Geometry: final body of the model. Coordinates: model frame, mm. A direction names the side the tool comes from. Coordinates: 2 decimals unless noted, no trailing zeros. Write each loop counter-clockwise with the first axis right and the second up, starting at its lowest first coordinate (ties: lowest second). Pieces come first, ordered by that corner, then holes.
from build123d import *

# Parameters (mm, degrees)
SKETCH1_W            = 68
SKETCH1_H            = 70
BOSS_EXTRUDE2_DEPTH  = 4
SKETCH2_W            = 13.5
SKETCH2_H            = 5
BOSS_EXTRUDE4_DEPTH  = 22
SKETCH3_R            = 2
CUT_EXTRUDE1_DEPTH   = 10
SKETCH4_W            = 5
SKETCH4_H            = 25.69
BOSS_EXTRUDE5_DEPTH  = 15
SKETCH5_R            = 1.3
CUT_EXTRUDE2_DEPTH   = 6
SKETCH6_W            = 68
SKETCH6_H            = 4
BOSS_EXTRUDE6_DEPTH  = 10
BOSS_EXTRUDE7_DEPTH  = 22
SKETCH8_W            = 3
SKETCH8_H            = 26
BOSS_EXTRUDE8_DEPTH  = 22
BOSS_EXTRUDE9_DEPTH  = 22
SKETCH12_W           = 3
SKETCH12_H           = 1
CUT_EXTRUDE5_DEPTH   = 7
SKETCH13_W           = 68
SKETCH13_H           = 26
SKETCH13_H_2         = 15
BOSS_EXTRUDE12_DEPTH = 8
SKETCH19_W           = 6
SKETCH19_H           = 61
CUT_EXTRUDE8_DEPTH   = 22
SKETCH20_W           = 3
SKETCH20_H           = 3
BOSS_EXTRUDE13_DEPTH = 22
SKETCH21_R           = 2.5
CUT_EXTRUDE9_DEPTH   = 22
SKETCH22_R           = 5.004310541
SKETCH22_R_2         = 5.00398022
SKETCH22_R_3         = 4.995044229
SKETCH22_R_4         = 4.998284189
CUT_EXTRUDE10_DEPTH  = 6
SKETCH24_W           = 3
SKETCH24_H           = 3
BOSS_EXTRUDE14_DEPTH = 22
SKETCH26_R           = 1.2
CUT_EXTRUDE11_DEPTH  = 5
SKETCH27_R           = 2.5
CUT_EXTRUDE13_DEPTH  = 10
FILLET2_R            = 2.5


with BuildPart() as part:
    # Sketch1 → Boss-Extrude2 (new body)
    with BuildSketch(Plane(origin=(0, 0, 0), x_dir=(1, 0, 0), z_dir=(0, 1, 0))):
        with Locations((34, -35)):
            Rectangle(SKETCH1_W, SKETCH1_H)
    extrude(amount=BOSS_EXTRUDE2_DEPTH)

    # Sketch2 → Boss-Extrude4 (add)
    with BuildSketch(Plane(origin=(0, 0, 0), x_dir=(-1, 0, 0), z_dir=(0, -1, 0))):
        with Locations((-6.75, -13.5)):
            Rectangle(SKETCH2_W, SKETCH2_H)
        with Locations((-61.25, -13.5)):
            Rectangle(SKETCH2_W, SKETCH2_H)
    extrude(amount=BOSS_EXTRUDE4_DEPTH)

    # Sketch3 → Cut-Extrude1 (cut)
    with BuildSketch(Plane(origin=(0, 0, 11), x_dir=(-1, 0, 0), z_dir=(0, 0, -1))):
        with Locations((-59.07, -14.83)):
            Circle(SKETCH3_R)
        with Locations((-59.07, -4.71)):
            Circle(SKETCH3_R)
        with Locations((-8.93, -14.83)):
            Circle(SKETCH3_R)
        with Locations((-8.93, -4.71)):
            Circle(SKETCH3_R)
    extrude(amount=-CUT_EXTRUDE1_DEPTH, mode=Mode.SUBTRACT)

    # Sketch4 → Boss-Extrude5 (add)
    with BuildSketch(Plane(origin=(0, 0, 0), x_dir=(-1, 0, 0), z_dir=(0, -1, 0))):
        with Locations((-2.5, -54.845)):
            Rectangle(SKETCH4_W, SKETCH4_H)
        with Locations((-45.65, -54.845)):
            Rectangle(SKETCH4_W, SKETCH4_H)
    extrude(amount=BOSS_EXTRUDE5_DEPTH)

    # Sketch5 → Cut-Extrude2 (cut)
    with BuildSketch(Plane(origin=(0, -15, 0), x_dir=(-1, 0, 0), z_dir=(0, -1, 0))):
        with Locations((-2.3, -65.24)):
            Circle(SKETCH5_R)
        with Locations((-2.3, -44.45)):
            Circle(SKETCH5_R)
        with Locations((-45.85, -65.24)):
            Circle(SKETCH5_R)
        with Locations((-45.85, -44.45)):
            Circle(SKETCH5_R)
    extrude(amount=-CUT_EXTRUDE2_DEPTH, mode=Mode.SUBTRACT)

    # Sketch6 → Boss-Extrude6 (add)
    with BuildSketch(Plane.XY.offset(70)):
        with Locations((34, 2)):
            Rectangle(SKETCH6_W, SKETCH6_H)
    extrude(amount=BOSS_EXTRUDE6_DEPTH)

    # Sketch7 → Boss-Extrude7 (add)
    with BuildSketch(Plane(origin=(0, 0, 0), x_dir=(-1, 0, 0), z_dir=(0, -1, 0))):
        Polygon((0, -80), (0, -67.69), (-3, -67.69), (-3, -77), (-59, -77), (-59, -16), (-68, -16), (-68, -80), align=None)
    extrude(amount=BOSS_EXTRUDE7_DEPTH)

    # Sketch8 → Boss-Extrude8 (add)
    with BuildSketch(Plane(origin=(0, 0, 0), x_dir=(-1, 0, 0), z_dir=(0, -1, 0))):
        with Locations((-1.5, -29)):
            Rectangle(SKETCH8_W, SKETCH8_H)
    extrude(amount=BOSS_EXTRUDE8_DEPTH)

    # Sketch9 → Boss-Extrude9 (add)
    with BuildSketch(Plane.XZ):
        Polygon((68, 11), (68, 0), (65, 0), (65, 3), (65, 11), align=None)
        Polygon((0, 11), (0, 0), (3, 0), (3, 3), (3, 11), align=None)
    extrude(amount=BOSS_EXTRUDE9_DEPTH)

    # Sketch12 → Cut-Extrude5 (cut)
    with BuildSketch(Plane(origin=(0, -22, 0), x_dir=(-1, 0, 0), z_dir=(0, -1, 0))):
        with Locations((-1.5, -41.5)):
            Rectangle(SKETCH12_W, SKETCH12_H)
        with Locations((-1.5, -68.19)):
            Rectangle(SKETCH12_W, SKETCH12_H)
    extrude(amount=-CUT_EXTRUDE5_DEPTH, mode=Mode.SUBTRACT)

    # Sketch13 → Boss-Extrude12 (add)
    with BuildSketch(Plane(origin=(0, 4, 0), x_dir=(1, 0, 0), z_dir=(0, 1, 0))):
        with Locations((34, -24)):
            Rectangle(SKETCH13_W, SKETCH13_H)
        with Locations((34, -72.5)):
            Rectangle(SKETCH13_W, SKETCH13_H_2)
    extrude(amount=BOSS_EXTRUDE12_DEPTH)

    # Sketch19 → Cut-Extrude8 (cut)
    with BuildSketch(Plane(origin=(0, -22, 0), x_dir=(-1, 0, 0), z_dir=(0, -1, 0))):
        with Locations((-62, -46.5)):
            Rectangle(SKETCH19_W, SKETCH19_H)
    extrude(amount=-CUT_EXTRUDE8_DEPTH, mode=Mode.SUBTRACT)

    # Sketch20 → Boss-Extrude13 (add)
    with BuildSketch(Plane.XZ):
        with Locations((4.5, 17.5)):
            Rectangle(SKETCH20_W, SKETCH20_H)
        with Locations((63.5, 17.5)):
            Rectangle(SKETCH20_W, SKETCH20_H)
    extrude(amount=BOSS_EXTRUDE13_DEPTH)

    # Sketch21 → Cut-Extrude9 (cut)
    with BuildSketch(Plane(origin=(0, 0, 0), x_dir=(-1, 0, 0), z_dir=(0, -1, 0))):
        with Locations((-8.5, -26)):
            Circle(SKETCH21_R)
        with Locations((-12, -71.5)):
            Circle(SKETCH21_R)
        with Locations((-56, -71.5)):
            Circle(SKETCH21_R)
        with Locations((-59.5, -26)):
            Circle(SKETCH21_R)
    extrude(amount=-CUT_EXTRUDE9_DEPTH, mode=Mode.SUBTRACT)

    # Sketch22 → Cut-Extrude10 (cut)
    with BuildSketch(Plane(origin=(0, 0, 0), x_dir=(-1, 0, 0), z_dir=(0, -1, 0))):
        with Locations((-12, -71.5)):
            Circle(SKETCH22_R)
        with Locations((-8.5, -26)):
            Circle(SKETCH22_R_2)
        with Locations((-59.5, -26)):
            Circle(SKETCH22_R_3)
        with Locations((-56, -71.5)):
            Circle(SKETCH22_R_4)
    extrude(amount=-CUT_EXTRUDE10_DEPTH, mode=Mode.SUBTRACT)

    # Sketch24 → Boss-Extrude14 (add)
    with BuildSketch(Plane(origin=(0, 0, 0), x_dir=(-1, 0, 0), z_dir=(0, -1, 0))):
        with Locations((-4.5, -75.5)):
            Rectangle(SKETCH24_W, SKETCH24_H)
        with Locations((-63.5, -75.5)):
            Rectangle(SKETCH24_W, SKETCH24_H)
    extrude(amount=BOSS_EXTRUDE14_DEPTH)

    # Sketch26 → Cut-Extrude11 (cut)
    with BuildSketch(Plane(origin=(0, -22, 0), x_dir=(-1, 0, 0), z_dir=(0, -1, 0))):
        with Locations((-65, -77)):
            Circle(SKETCH26_R)
        with Locations((-3, -77)):
            Circle(SKETCH26_R)
        with Locations((-65, -16)):
            Circle(SKETCH26_R)
        with Locations((-3, -16)):
            Circle(SKETCH26_R)
    extrude(amount=-CUT_EXTRUDE11_DEPTH, mode=Mode.SUBTRACT)

    # Sketch27 → Cut-Extrude13 (cut)
    with BuildSketch(Plane(origin=(0, 0, 0), x_dir=(-1, 0, 0), z_dir=(0, -1, 0))):
        with Locations((-36.8, -42)):
            Circle(SKETCH27_R)
        with Locations((-30.45, -42)):
            Circle(SKETCH27_R)
        with Locations((-24.075, -42)):
            Circle(SKETCH27_R)
        with Locations((-17.7, -42)):
            Circle(SKETCH27_R)
        with Locations((-11.35, -42)):
            Circle(SKETCH27_R)
        with Locations((-11.35, -48.4225)):
            Circle(SKETCH27_R)
        with Locations((-17.7, -48.4225)):
            Circle(SKETCH27_R)
        with Locations((-24.075, -48.4225)):
            Circle(SKETCH27_R)
        with Locations((-30.45, -48.4225)):
            Circle(SKETCH27_R)
        with Locations((-36.8, -48.4225)):
            Circle(SKETCH27_R)
        with Locations((-36.8, -54.845)):
            Circle(SKETCH27_R)
        with Locations((-36.8, -61.2675)):
            Circle(SKETCH27_R)
        with Locations((-30.45, -54.845)):
            Circle(SKETCH27_R)
        with Locations((-30.45, -61.2675)):
            Circle(SKETCH27_R)
        with Locations((-24.075, -54.845)):
            Circle(SKETCH27_R)
        with Locations((-24.075, -61.2675)):
            Circle(SKETCH27_R)
        with Locations((-17.7, -54.845)):
            Circle(SKETCH27_R)
        with Locations((-17.7, -61.2675)):
            Circle(SKETCH27_R)
        with Locations((-11.35, -54.845)):
            Circle(SKETCH27_R)
        with Locations((-11.35, -61.2675)):
            Circle(SKETCH27_R)
    extrude(amount=-CUT_EXTRUDE13_DEPTH, mode=Mode.SUBTRACT)

    # Fillet2
    fillet2_edges = [part.edges().sort_by_distance(p)[0] for p in [
        (0, -5, 80),
        (68, -5, 80),
        (0, -9, 0),
        (68, -9, 0),
    ]]
    fillet(fillet2_edges, radius=FILLET2_R)


solid = part.part
Item 1: Section B-B, the plane z = 26. Output: boundary loops of the cut face in (x, y), plus the area to 3 significant figures.
Derived:
outline: (0, -22) - (3, -22) - (3, 0) - (3.5, 0) - (3.5, 6) - (6, 6) - (6, 12) - (0, 12) - close; (11, 6) - (13.5, 6) - (13.5, 0) - (54.5, 0) - (54.5, 6) - (57, 6) - (57, 12) - (11, 12) - close; (62, 6) - (64.5, 6) - (64.5, 0) - (65, 0) - (65, -22) - (68, -22) - (68, 12) - (62, 12) - close
area: 768 mm2
Item 2: Material intervals for probe 1 along X at (y, z) = (0.95, 42) (3 decimals); probe 2 along X at (y, z) = (1.9, 26); probe 3 along Z at (x, y) = (7, -2), sorted ascending.
Derived:
probe 1: x = 0 to 8.85, 13.85 to 15.2, 20.2 to 21.575, 26.575 to 27.95, 32.95 to 34.3, 39.3 to 68
probe 2: x = 0 to 3.5, 13.5 to 54.5, 64.5 to 68
probe 3: z = 11 to 16, 77 to 80
Item 3: Pull-direction query (Z, two-part tool) for faces 1 (the cylindrical face through (13.085, 2.958, 76.385)), 2 (the cylindrical face through (0.713, -4.762, 79.248)), 3 (the cylindrical face through (2.58, -12.04, 45.72)), 4 (the flat face through (3, -11, 5)); classes: released by +Z, released by -Z, zero draft, split by the parting line, or undercut.
Derived:
face 1: undercut
face 2: released by +Z
face 3: undercut
face 4: zero draft
Item 4: Set-up query: faces 5 (the flat face through (43.15, -7, 55)), 6 (the flat face through (65, -17, 16)), 7 (the cylindrical face through (58, 9, 24)), 8 (the cylindrical face through (61.068, -4.622, 13.465)). Return all of +Z, -Z, +X, -X, +Y, -Y with unobstructed straight access to the full face (end or side cutting, diameter ignored); none if empty.
Derived:
face 5: -Z, -Y
face 6: -Y
face 7: +Y, -Y
face 8: -Z
Item 5: Section C-C, the plane x = 56. Output: boundary loops of the cut face in (y, z), plus the area to 3 significant figures.
Derived:
outline: (-22, 11) - (0, 11) - (0, 0) - (4, 0) - (4, 11) - (12, 11) - (12, 37) - (4, 37) - (4, 65) - (12, 65) - (12, 69) - (6, 69) - (6, 66.5) - (0, 66.5) - (0, 29.56) - (6, 29.56) - (6, 22.44) - (0, 22.44) - (0, 16) - (-22, 16) - close; (-22, 77) - (0, 77) - (0, 76.5) - (6, 76.5) - (6, 74) - (12, 74) - (12, 80) - (-22, 80) - close
area: 691 mm2
Item 6: Section D-D, the plane z = 13.5. Output: boundary loops of the cut face in (x, y).
Derived:
outline: (0, -22) - (13.5, -22) - (13.5, 0) - (54.5, 0) - (54.5, -22) - (68, -22) - (68, 12) - (0, 12) - close; hole circle Ø4 at (8.93, -14.83); hole circle Ø4 at (8.93, -4.71); hole circle Ø4 at (59.07, -14.83); hole circle Ø4 at (59.07, -4.71)
Item 7: Section A-A, the plane x = 30.45. Output: boundary loops of the cut face in (y, z) (1 decimal), plus the area to 3 significant figures.
Derived:
outline: (-22, 77) - (0, 77) - (0, 63.8) - (4, 63.8) - (4, 65) - (12, 65) - (12, 80) - (-22, 80) - close; (0, 0) - (4, 0) - (4, 11) - (12, 11) - (12, 37) - (4, 37) - (4, 39.5) - (0, 39.5) - close; (0, 44.5) - (4, 44.5) - (4, 45.9) - (0, 45.9) - close; (0, 50.9) - (4, 50.9) - (4, 52.3) - (0, 52.3) - close; (0, 57.3) - (4, 57.3) - (4, 58.8) - (0, 58.8) - close
area: 634 mm2
Item 8: Pin query (flat end, axial travel): pin 1 (8 mm diameter, centred on x = 11.35, z = 42, fed in from -Y); pin 2 (1.5 mm diameter, centred on x = 13.5, z = 8, fed in from +Y); pin 3 (4.5 mm diameter, centred on x = 8.5, z = 26, fed in from +Y); pin 4 (0.7 mm diameter, centred on x = 65, z = 77, fed in from -Y). Return the tip coordinate at first contact, or that it passes through.
Derived:
pin 1: stops at y = 0
pin 2: stops at y = 4
pin 3: passes through
pin 4: stops at y = -17
